from build123d import *

# Parameters (mm, degrees)
SKETCH1_W           = 41.91
SKETCH1_H           = 10.16
BOSS_EXTRUDE1_DEPTH = 3.683
SKETCH2_2_R         = 1.174037675
CUT_EXTRUDE1_DEPTH  = 4.683


with BuildPart() as part:
    # Sketch1 → Boss-Extrude1 (new body)
    with BuildSketch(Plane(origin=(0, 0, 0), x_dir=(1, 0, 0), z_dir=(0, 1, 0))):
        Rectangle(SKETCH1_W, SKETCH1_H)
    extrude(amount=BOSS_EXTRUDE1_DEPTH)

    # Sketch2<2> → Cut-Extrude1 (cut, through all)
    with BuildSketch(Plane.XZ):
        with Locations((-13.462, 0)):
            Circle(SKETCH2_2_R)
        with Locations((-8.128, 0)):
            Circle(SKETCH2_2_R)
        with Locations((8.128, 0)):
            Circle(SKETCH2_2_R)
        with Locations((13.462, 0)):
            Circle(SKETCH2_2_R)
    extrude(amount=-CUT_EXTRUDE1_DEPTH, mode=Mode.SUBTRACT)


solid = part.part
Geometry: final body of the model. Coordinates: model frame, mm. Give positions to 0.01 mm unless a question says otherwise; leave off trailing zeros. Write each loop counter-clockwise with the first axis right and the second up, starting at its lowest first coordinate (ties: lowest second). Pieces come first, ordered by that corner, then holes. Notation, with made-up numbers: (42, -0.75) -> (91, -0.75) arc R18 ccw to (91, 6.25) -> close; hole circle Ø9 at (10, 77.25). An arc over 180 degrees is marked (long way). Answer as a JSON object with one key per item and string values.
1. Mould query, pull axis Z, two halves, no side actions, for faces 1 (the flat face through (20.955, 2, 0)), 2 (the flat face through (0, 2, -5.08)), 3 (the cylindrical face through (14.547, 1.816, -0.45)), 4 (the flat face through (0, 2, 5.08)). Classes: pulls with the +Z half, pulls with the -Z half, needs draft (parallel to the pull), parting line crosses it, or undercut.
Ans:
{"face 1": "needs draft", "face 2": "pulls with the -Z half", "face 3": "undercut", "face 4": "pulls with the +Z half"}
2. Ray query, probe 1 along X at (y, z) = (1.1, -1) (3 decimals); probe 2 along Z at (x, y) = (8, 0.45); probe 3 along X at (y, z) = (0.3, -0.25) (3 decimals). Return the intervals inside material, ascending. Write a range as from..to.
Ans:
{"probe 1": "x = -20.955..-14.077, -12.847..-8.743, -7.513..7.513, 8.743..12.847, 14.077..20.955", "probe 2": "z = -5.08..-1.17, 1.17..5.08", "probe 3": "x = -20.955..-14.609, -12.315..-9.275, -6.981..6.981, 9.275..12.315, 14.609..20.955"}
3. Contact query for a flat-ended pin moving along its axis: pin 1 (1.9 mm diameter, centred on x = -8.128, z = 0, fed in from +Y). Output: stop coordinate, or through.
Ans:
{"pin 1": "passes through"}
4. Cut plane B-B on z = 0. Output: boundary loops of the cut face in (x, y) (3 decimals), and give its area (3 significant figures).
Ans:
{"outline": "(-20.955, 0) -> (-14.636, 0) -> (-14.636, 3.683) -> (-20.955, 3.683) -> close; (-12.288, 0) -> (-9.302, 0) -> (-9.302, 3.683) -> (-12.288, 3.683) -> close; (-6.954, 0) -> (6.954, 0) -> (6.954, 3.683) -> (-6.954, 3.683) -> close; (9.302, 0) -> (12.288, 0) -> (12.288, 3.683) -> (9.302, 3.683) -> close; (14.636, 0) -> (20.955, 0) -> (20.955, 3.683) -> (14.636, 3.683) -> close", "area": "120 mm^2"}
5. Cut plane A-A on y = 1.8. Output: boundary loops of the cut face in (x, z) (3 decimals), and give its area (3 significant figures).
Ans:
{"outline": "(-20.955, -5.08) -> (20.955, -5.08) -> (20.955, 5.08) -> (-20.955, 5.08) -> close; hole circle Ø2.348 at (-13.462, 0); hole circle Ø2.348 at (-8.128, 0); hole circle Ø2.348 at (8.128, 0); hole circle Ø2.348 at (13.462, 0)", "area": "408 mm^2"}
